Can you work these out from the model? Positions are in its coordinate system, mm. A direction names the side the tool comes from. Coordinates: 2 decimals unless noted, no trailing zeros. Loops run counter-clockwise (first coordinate to the right, second up) from the corner with the lowest first, then second, coordinate; pieces in that order, holes last. Notation, with made-up numbers: (-3, -5.75) -> (1, -5.75) arc R12 ccw to (1, -1.75) -> close; hole circle Ø8 at (-40, -19.5). An arc over 180 degrees is marked (long way). Use one line per item in the form item = value. Start each with the question number.
(1) Thinking about a two-plate mould opening in Z: for faces 1 (the flat face through (10, 5.3, 50)), 2 (the flat face through (64.034, 3.779, 60.889)), which applies, released by +Z, released by -Z, zero draft, split by the parting line, or undercut?
(2) Imagine slicing it at D-D (z = 55). List the corners of the cut face in (x, y) for me, plus the area to 3 significant figures.
(3) Imagine slicing it at A-A (z = 35). List the corners of the cut face in (x, y) for me, plus the area to 3 significant figures.
(4) I'm going to push flat-ended pins straight in: pin 1 (3 mm diameter, centred on x = -32.5, z = 122.5, fed in from +Y); pin 2 (1.4 mm diameter, centred on y = 3, z = 89.5, fed in from -X); pin 3 (0.6 mm diameter, centred on x = 91, y = 4.5, fed in from -Z); pin 4 (1.5 mm diameter, centred on y = 3.5, z = 20, fed in from -X). Where does each tip first touch, or does it pass through?
(5) On a 3-axis mill with a long thin cutter (end or side, diameter ignored), from which of +Z, -Z, +X, -X, +Y, -Y can I reach the whole of each face in a straight line? I mean faces 3 (the flat face through (10, 2.3, 50)), 4 (the flat face through (-29.116, 3.779, 61.002)). Say none if no direction works.
(6) I need wall thicknesses on line 1 (Z direction, x = 5, y = 3.6); line 2 (Z direction, x = 66, y = 2.6); line 3 (X direction, y = 4.35, z = 109.5). Which ranges of each line are inside material? Lowest first, please. Write a range as [from, to].
(7) Imagine slicing it at C-C (z = 122.5). State how many separate pieces and enclosed holes the cut face has, plus the area to 3 significant figures.
(8) Imagine slicing it at B-B (x = 30). List the corners of the cut face in (y, z) for me, plus the area to 3 significant figures.
```python
from build123d import *

# Parameters (mm, degrees)
SKETCH_1_R          = 2
EXTRUDE_1_DEPTH     = 4
SKETCH_2_R          = 1.5
SKETCH_2_R_2        = 2
EXTRUDE_2_DEPTH     = 4
CUT_EXTRUDE_1_DEPTH = 174.943237868
FILLET_2_R          = 1
FILLET_3_R          = 1
CUT_EXTRUDE_START   = -12.7
CUT_EXTRUDE_2_DEPTH = 11
SKETCH_5_R          = 2
SKETCH_5_R_2        = 1.5
EXTRUDE_3_DEPTH     = 1.3


with BuildPart() as part:
    # 草图1 → 凸台-拉伸1 (new body)
    with BuildSketch(Plane(origin=(0, 0, 0), x_dir=(1, 0, 0), z_dir=(0, 1, 0))):
        Polygon((0, 0), (0, -110), (-62.5, -110), (-62.5, -130), (97.5, -130), (97.5, -110), (35, -110), (35, 0), align=None)
        with Locations(Location((5, -5, 0), (0, 0, 270))):
            Circle(SKETCH_1_R, mode=Mode.SUBTRACT)
        with Locations(Location((30, -5, 0), (0, 0, 270))):
            Circle(SKETCH_1_R, mode=Mode.SUBTRACT)
        with Locations(Location((5, -35, 0), (0, 0, 270))):
            Circle(SKETCH_1_R, mode=Mode.SUBTRACT)
        with Locations(Location((30, -35, 0), (0, 0, 270))):
            Circle(SKETCH_1_R, mode=Mode.SUBTRACT)
        with Locations(Location((-52.5, -122.5, 0), (0, 0, 270))):
            Circle(SKETCH_1_R, mode=Mode.SUBTRACT)
        with Locations(Location((-32.5, -122.5, 0), (0, 0, 270))):
            Circle(SKETCH_1_R, mode=Mode.SUBTRACT)
        with Locations(Location((-12.5, -122.5, 0), (0, 0, 270))):
            Circle(SKETCH_1_R, mode=Mode.SUBTRACT)
        with Locations(Location((7.5, -122.5, 0), (0, 0, 270))):
            Circle(SKETCH_1_R, mode=Mode.SUBTRACT)
        with Locations(Location((27.5, -122.5, 0), (0, 0, 270))):
            Circle(SKETCH_1_R, mode=Mode.SUBTRACT)
        with Locations(Location((47.5, -122.5, 0), (0, 0, 270))):
            Circle(SKETCH_1_R, mode=Mode.SUBTRACT)
        with Locations(Location((67.5, -122.5, 0), (0, 0, 270))):
            Circle(SKETCH_1_R, mode=Mode.SUBTRACT)
        with Locations(Location((87.5, -122.5, 0), (0, 0, 270))):
            Circle(SKETCH_1_R, mode=Mode.SUBTRACT)
    extrude(amount=EXTRUDE_1_DEPTH)

    # 草图2 → 凸台-拉伸2 (add)
    # profile 1 of 2: a face of its own
    with BuildSketch(Plane(origin=(0, 4, 0), x_dir=(1, 0, 0), z_dir=(0, 1, 0))):
        Polygon((0, -40), (0, -53), (-26.149225941, -56.891259047), (-32, -65), (-32, -110), (-41, -110), (-41, -70.637206461), (-69.401796613, -110), (-62.5, -110), (-62.5, -130), (-80.5, -130), (-80.5, -110), (-33.599955214, -45), align=None)
        with Locations(Location((-35, -65, 0), (0, 0, 270))):
            Circle(SKETCH_2_R, mode=Mode.SUBTRACT)
        with Locations(Location((-35, -75, 0), (0, 0, 270))):
            Circle(SKETCH_2_R, mode=Mode.SUBTRACT)
        with Locations(Location((-72.5, -122.5, 0), (0, 0, 270))):
            Circle(SKETCH_2_R_2, mode=Mode.SUBTRACT)
    # profile 2 of 2: a face of its own
    with BuildSketch(Plane(origin=(0, 4, 0), x_dir=(1, 0, 0), z_dir=(0, 1, 0))):
        Polygon((67, -65), (67, -110), (76, -110), (76, -70.637206461), (104.401796613, -110), (97.5, -110), (97.5, -130), (115.5, -130), (115.5, -110), (68.599955214, -45), (35, -40), (35, -53), (61.149225941, -56.891259047), align=None)
        with Locations(Location((70, -65, 0), (0, 0, 270))):
            Circle(SKETCH_2_R, mode=Mode.SUBTRACT)
        with Locations(Location((70, -75, 0), (0, 0, 270))):
            Circle(SKETCH_2_R, mode=Mode.SUBTRACT)
        with Locations(Location((107.5, -122.5, 0), (0, 0, 270))):
            Circle(SKETCH_2_R_2, mode=Mode.SUBTRACT)
    extrude(amount=-EXTRUDE_2_DEPTH)

    # 草图3 → 切除-拉伸1 (cut, through all)
    with BuildSketch(Plane(origin=(0, 4, 0), x_dir=(1, 0, 0), z_dir=(0, 1, 0))):
        Polygon((0, -53), (35, -53), (35, -110), (60.5, -110), (60.5, -130), (-25.5, -130), (-25.5, -110), (0, -110), align=None)
    extrude(amount=-CUT_EXTRUDE_1_DEPTH, mode=Mode.SUBTRACT)

    # 圆角2
    fillet_2_edges = [part.edges().sort_by_distance(p)[0] for p in [
        (76, 2, 70.637206461),
        (104.401796613, 2, 110),
        (76, 2, 110),
        (-41, 2, 70.637206461),
        (-41, 2, 110),
        (-69.401796613, 2, 110),
    ]]
    fillet(fillet_2_edges, radius=FILLET_2_R)

    # 圆角3
    fillet_3_edges = [part.edges().sort_by_distance(p)[0] for p in [
        (115.5, 2, 130),
        (115.5, 2, 110),
        (68.599955214, 2, 45),
        (60.5, 2, 110),
        (60.5, 2, 130),
        (-25.5, 2, 130),
        (-25.5, 2, 110),
        (-33.599955214, 2, 45),
        (-80.5, 2, 110),
        (-80.5, 2, 130),
    ]]
    fillet(fillet_3_edges, radius=FILLET_3_R)

    # 草图4 → 切除-拉伸2 (cut)
    with BuildSketch(Plane(origin=(0, 4, 0), x_dir=(1, 0, 0), z_dir=(0, 1, 0)).offset(CUT_EXTRUDE_START)):
        with BuildLine():
            Line((0, -40), (-33.182912111, -44.937939932))
            ThreePointArc((-33.182912111, -44.937939932), (-33.555630957, -45.072825937), (-33.846665233, -45.341921875))
            Line((-33.846665233, -45.341921875), (-80.310942068, -109.737979661))
            ThreePointArc((-80.310942068, -109.737979661), (-80.451562417, -110.015650479), (-80.5, -110.323106112))
            Line((-80.5, -110.323106112), (-80.5, -129))
            ThreePointArc((-80.5, -129), (-80.207106781, -129.707106781), (-79.5, -130))
            Line((-79.5, -130), (-26.5, -130))
            ThreePointArc((-26.5, -130), (-25.792893219, -129.707106781), (-25.5, -129))
            Line((-25.5, -129), (-25.5, -111))
            ThreePointArc((-25.5, -111), (-25.792893219, -110.292893219), (-26.5, -110))
            Line((-26.5, -110), (-32, -110))
            Line((-32, -110), (-32, -65))
            Line((-32, -65), (-26.149225941, -56.891259047))
            Line((-26.149225941, -56.891259047), (0, -53))
            Line((0, -53), (35, -53))
            Line((35, -53), (61.149225941, -56.891259047))
            Line((61.149225941, -56.891259047), (67, -65))
            Line((67, -65), (67, -110))
            Line((67, -110), (61.5, -110))
            ThreePointArc((61.5, -110), (60.792893219, -110.292893219), (60.5, -111))
            Line((60.5, -111), (60.5, -129))
            ThreePointArc((60.5, -129), (60.792893219, -129.707106781), (61.5, -130))
            Line((61.5, -130), (114.5, -130))
            ThreePointArc((114.5, -130), (115.207106781, -129.707106781), (115.5, -129))
            Line((115.5, -129), (115.5, -110.323106112))
            ThreePointArc((115.5, -110.323106112), (115.451562417, -110.015650479), (115.310942068, -109.737979661))
            Line((115.310942068, -109.737979661), (68.846665233, -45.341921875))
            ThreePointArc((68.846665233, -45.341921875), (68.555630957, -45.072825937), (68.182912111, -44.937939932))
            Line((68.182912111, -44.937939932), (35, -40))
            Line((35, -40), (35, 0))
            Line((35, 0), (0, 0))
            Line((0, 0), (0, -40))
        make_face()
    extrude(amount=CUT_EXTRUDE_2_DEPTH, mode=Mode.SUBTRACT)

    # 草图5 → 凸台-拉伸3 (add)
    with BuildSketch(Plane(origin=(0, 4, 0), x_dir=(1, 0, 0), z_dir=(0, 1, 0))):
        with BuildLine():
            Line((0, -40), (-33.182912111, -44.937939932))
            ThreePointArc((-33.182912111, -44.937939932), (-33.555630957, -45.072825937), (-33.846665233, -45.341921875))
            Line((-33.846665233, -45.341921875), (-80.310942068, -109.737979661))
            ThreePointArc((-80.310942068, -109.737979661), (-80.451562417, -110.015650479), (-80.5, -110.323106112))
            Line((-80.5, -110.323106112), (-80.5, -129))
            ThreePointArc((-80.5, -129), (-80.207106781, -129.707106781), (-79.5, -130))
            Line((-79.5, -130), (-26.5, -130))
            ThreePointArc((-26.5, -130), (-25.792893219, -129.707106781), (-25.5, -129))
            Line((-25.5, -129), (-25.5, -111))
            ThreePointArc((-25.5, -111), (-25.792893219, -110.292893219), (-26.5, -110))
            Line((-26.5, -110), (-32, -110))
            Line((-32, -110), (-32, -65))
            Line((-32, -65), (-26.149225941, -56.891259047))
            Line((-26.149225941, -56.891259047), (0, -53))
            Line((0, -53), (35, -53))
            Line((35, -53), (61.149225941, -56.891259047))
            Line((61.149225941, -56.891259047), (67, -65))
            Line((67, -65), (67, -110))
            Line((67, -110), (61.5, -110))
            ThreePointArc((61.5, -110), (60.792893219, -110.292893219), (60.5, -111))
            Line((60.5, -111), (60.5, -129))
            ThreePointArc((60.5, -129), (60.792893219, -129.707106781), (61.5, -130))
            Line((61.5, -130), (114.5, -130))
            ThreePointArc((114.5, -130), (115.207106781, -129.707106781), (115.5, -129))
            Line((115.5, -129), (115.5, -110.323106112))
            ThreePointArc((115.5, -110.323106112), (115.451562417, -110.015650479), (115.310942068, -109.737979661))
            Line((115.310942068, -109.737979661), (68.846665233, -45.341921875))
            ThreePointArc((68.846665233, -45.341921875), (68.555630957, -45.072825937), (68.182912111, -44.937939932))
            Line((68.182912111, -44.937939932), (35, -40))
            Line((35, -40), (35, 0))
            Line((35, 0), (0, 0))
            Line((0, 0), (0, -40))
        make_face()
        with Locations(Location((30, -5, 0), (0, 0, 270))):
            Circle(SKETCH_5_R, mode=Mode.SUBTRACT)
        with Locations(Location((30, -35, 0), (0, 0, 270))):
            Circle(SKETCH_5_R, mode=Mode.SUBTRACT)
        with Locations(Location((-32.5, -122.5, 0), (0, 0, 270))):
            Circle(SKETCH_5_R, mode=Mode.SUBTRACT)
        with Locations(Location((87.5, -122.5, 0), (0, 0, 270))):
            Circle(SKETCH_5_R, mode=Mode.SUBTRACT)
        with Locations(Location((-72.5, -122.5, 0), (0, 0, 270))):
            Circle(SKETCH_5_R, mode=Mode.SUBTRACT)
        with Locations(Location((-35, -65, 0), (0, 0, 270))):
            Circle(SKETCH_5_R_2, mode=Mode.SUBTRACT)
        with Locations(Location((-35, -75, 0), (0, 0, 270))):
            Circle(SKETCH_5_R_2, mode=Mode.SUBTRACT)
        with Locations(Location((107.5, -122.5, 0), (0, 0, 270))):
            Circle(SKETCH_5_R, mode=Mode.SUBTRACT)
        with Locations(Location((70, -75, 0), (0, 0, 270))):
            Circle(SKETCH_5_R_2, mode=Mode.SUBTRACT)
        with Locations(Location((70, -65, 0), (0, 0, 270))):
            Circle(SKETCH_5_R_2, mode=Mode.SUBTRACT)
        with Locations(Location((67.5, -122.5, 0), (0, 0, 270))):
            Circle(SKETCH_5_R, mode=Mode.SUBTRACT)
        with Locations(Location((-52.5, -122.5, 0), (0, 0, 270))):
            Circle(SKETCH_5_R, mode=Mode.SUBTRACT)
        with Locations(Location((5, -35, 0), (0, 0, 270))):
            Circle(SKETCH_5_R, mode=Mode.SUBTRACT)
        with Locations(Location((5, -5, 0), (0, 0, 270))):
            Circle(SKETCH_5_R, mode=Mode.SUBTRACT)
        with BuildLine():
            Line((102.447123753, -110), (77, -110))
            ThreePointArc((77, -110), (76.292893219, -109.707106781), (76, -109))
            Line((76, -109), (76, -73.732164937))
            ThreePointArc((76, -73.732164937), (76.692544367, -72.78060252), (77.810942068, -73.147038486))
            Line((77.810942068, -73.147038486), (103.258065821, -108.414873549))
            ThreePointArc((103.258065821, -108.414873549), (103.337383954, -109.455452275), (102.447123753, -110))
        make_face(mode=Mode.SUBTRACT)
        with BuildLine():
            Line((-41, -73.732164937), (-41, -109))
            ThreePointArc((-41, -109), (-41.292893219, -109.707106781), (-42, -110))
            Line((-42, -110), (-67.447123753, -110))
            ThreePointArc((-67.447123753, -110), (-68.337383954, -109.455452275), (-68.258065821, -108.414873549))
            Line((-68.258065821, -108.414873549), (-42.810942068, -73.147038486))
            ThreePointArc((-42.810942068, -73.147038486), (-41.692544367, -72.78060252), (-41, -73.732164937))
        make_face(mode=Mode.SUBTRACT)
    extrude(amount=EXTRUDE_3_DEPTH)


solid = part.part
```
Worked out:
q1.face_1 = zero draft
q1.face_2 = undercut
q2.outline = (-40.82, 2.3) -> (-13.44, 2.3) -> (-13.44, 5.3) -> (-40.82, 5.3) -> close; (48.44, 2.3) -> (75.82, 2.3) -> (75.82, 5.3) -> (48.44, 5.3) -> close
q2.area = 164 mm2
q3.outline = (0, 2.3) -> (3, 2.3) -> (3, 5.3) -> (0, 5.3) -> close; (7, 2.3) -> (28, 2.3) -> (28, 5.3) -> (7, 5.3) -> close; (32, 2.3) -> (35, 2.3) -> (35, 5.3) -> (32, 5.3) -> close
q3.area = 81.0 mm2
q4.pin_1 = through
q4.pin_2 = -66.21
q4.pin_3 = 75.63
q4.pin_4 = 0
q5.face_3 = +Z, -Z, +X, -X, -Y
q5.face_4 = +Y, -Y
q6.line_1 = [0, 3], [7, 33], [37, 53]
q6.line_2 = [44.61, 63.61], [110, 121.18], [123.82, 130]
q6.line_3 = [-80.14, -68.31], [-41.13, -32], [67, 76.13], [103.31, 115.14]
q7.separate_pieces = 8
q7.enclosed_holes = 0
q7.area = 258 mm2
q8.outline = (2.3, 0) -> (5.3, 0) -> (5.3, 3) -> (2.3, 3) -> close; (2.3, 7) -> (5.3, 7) -> (5.3, 33) -> (2.3, 33) -> close; (2.3, 37) -> (5.3, 37) -> (5.3, 53) -> (2.3, 53) -> close
q8.area = 135 mm2
